Could you check a few things on this drawing? It's one solid part, dimensions in mm from its lowest x, y, z. A direction names the side the tool comes from. Round coordinates to 2 decimals unless told otherwise and drop trailing zeros. Order: outer loops, then holes, each group sorted by start corner. A loop starts at its lowest first (then second) coordinate and runs counter-clockwise, first axis right, second up. Notation, with made-up numbers: (-7, 84) -> (3, 84) arc R30 cw to (3, 117) -> close; hole circle Ø11 at (-38.75, 26.5). An arc over 180 degrees is marked (long way). Use a Markdown table: item, result. Add a question column.
(1) If I drill on probe 1 along Y at (x, z) = (10, 9.5); probe 2 along Z at (x, y) = (103.5, 31); probe 3 along X at (y, z) = (94, 5), over which ranges is the centre line in solid material (lowest first)?
(2) I want a section at C-C, the plane y = 50. Please give me the cut outline in (x, z).
(3) I want a section at B-B, the plane y = 90. Please give me the cut outline in (x, z).
(4) On a 3-axis mill with a long thin cutter (end or side, diameter ignored), from which of +Z, -Z, +X, -X, +Y, -Y can I reach the whole of each face in a straight line? I mean the marked faces 1 and 2. Say none if no direction works.
(5) I want a section at D-D, the plane x = 75. Please give me the cut outline in (y, z), then the cut area to 4 significant figures.
(6) I'm going to push flat-ended pins straight in: P1, Ø6, axis at x = 15.5, y = 87, coming from the +Z side; P2, Ø9, axis at x = 10, y = 90, coming from the -Z side. Where does each tip first touch, or does it pass through?
(7) I want a section at A-A, the plane x = 10. Please give me the cut outline in (y, z).
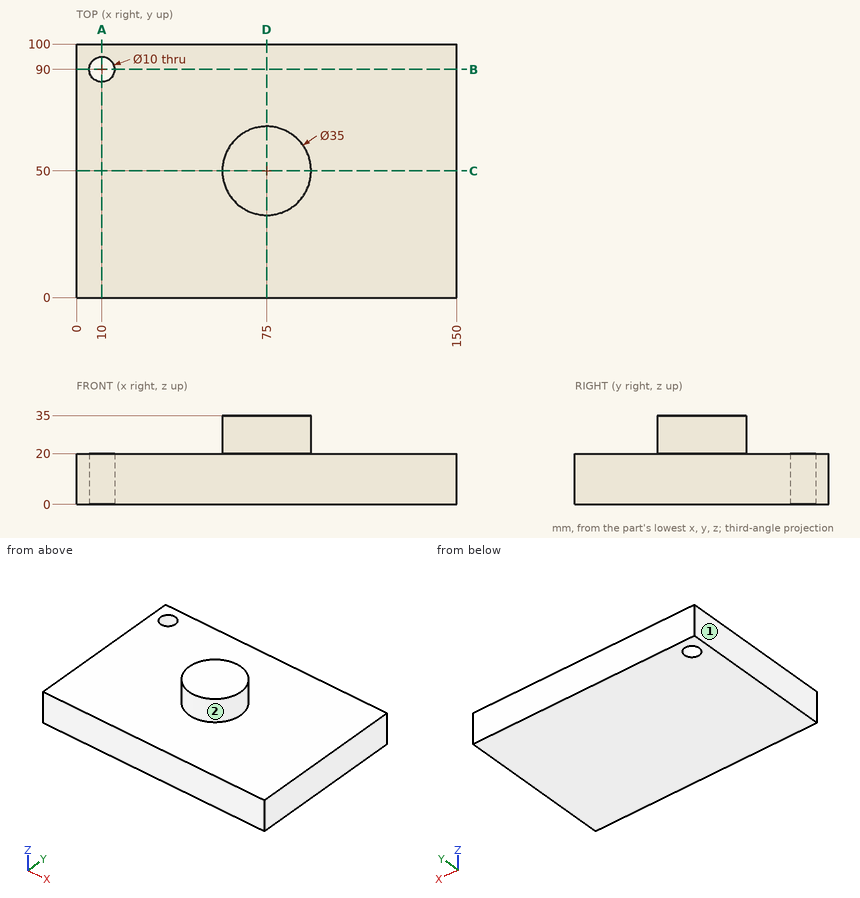
Taken from the geometry:
| question | item | result |
|---|---|---|
| 1 | probe 1 | y = 0 to 85, 95 to 100 |
| 1 | probe 2 | z = 0 to 20 |
| 1 | probe 3 | x = 0 to 7, 13 to 150 |
| 2 | outline | (0, 0) -> (150, 0) -> (150, 20) -> (92.5, 20) -> (92.5, 35) -> (57.5, 35) -> (57.5, 20) -> (0, 20) -> close |
| 3 | outline | (0, 0) -> (5, 0) -> (5, 20) -> (0, 20) -> close; (15, 0) -> (150, 0) -> (150, 20) -> (15, 20) -> close |
| 4 | face 1 | +Z, -Z, -X, +Y, -Y |
| 4 | face 2 | +Z |
| 5 | outline | (0, 0) -> (100, 0) -> (100, 20) -> (67.5, 20) -> (67.5, 35) -> (32.5, 35) -> (32.5, 20) -> (0, 20) -> close |
| 5 | area | 2,525 mm2 |
| 6 | P1 | stops at z = 20 |
| 6 | P2 | passes through |
| 7 | outline | (0, 0) -> (85, 0) -> (85, 20) -> (0, 20) -> close; (95, 0) -> (100, 0) -> (100, 20) -> (95, 20) -> close |
